from build123d import *

# Parameters (mm, degrees)
BOSS_EXTRUDE1_DEPTH = 38.1


with BuildPart() as part:
    # Sketch1 → Boss-Extrude1 (new body)
    with BuildSketch(Plane.XY):
        with BuildLine():
            Line((88.9, -50.8), (88.9, 50.8))
            ThreePointArc((88.9, 50.8), (57.095135122, 42.185130239), (25.4, 51.195336702))
            ThreePointArc((25.4, 51.195336702), (-57.15, 0), (25.4, -51.195336702))
            ThreePointArc((25.4, -51.195336702), (57.095135122, -42.185130239), (88.9, -50.8))
        make_face()
        with BuildLine():
            ThreePointArc((82.55, -40.628164989), (54.413891048, -35.903084421), (26.818032813, -43.144328898))
            ThreePointArc((26.818032813, -43.144328898), (24.611630749, -44.439932852), (22.342791686, -45.622797587))
            ThreePointArc((22.342791686, -45.622797587), (-50.735562995, 2.557859955), (26.818032813, 43.144328898))
            ThreePointArc((26.818032813, 43.144328898), (54.413891048, 35.903084421), (82.55, 40.628164989))
            Line((82.55, 40.628164989), (82.55, -40.628164989))
        make_face(mode=Mode.SUBTRACT)
    extrude(amount=BOSS_EXTRUDE1_DEPTH)


solid = part.part
Verification items for the finished model (mm, model axes). A direction names the side the tool comes from. Give positions to 0.01 mm unless a question says otherwise; leave off trailing zeros. Order: outer loops, then holes, each group sorted by start corner. A loop starts at its lowest first (then second) coordinate and runs counter-clockwise, first axis right, second up. Notation, with made-up numbers: M -12,-21.5 L 17,-21.5 A9 ccw 17,-16.5 Z; hole C 83,28.25 d9. An arc over 180 degrees is marked long. Use one line per item in the form item = value. Start each with the question number.
Q1. Section check B-B (x = 0). Enter the section's corners in (y, z).
Q2. Scan lines: line 1 along Y through (x, z) = (0, 8); line 2 along X through (y, z) = (3, 24); line 3 along Y through (x, z) = (67.5, 19.5). Record each from-to range of solid material in increasing order. Write a range as [from, to].
Q3. Access from +Z, -Z, +X, -X, +Y, -Y to the whole of each face (thin tool, end or side, straight path). Record for faces 4 (the cylindrical face through (56.63, -42.19, 18.78)), 5 (the flat face through (82.55, 1, 19)).
Q4. Section check A-A (y = 0). Enter the section's corners in (x, z), then the cut area to 3 significant figures.
Q5. Section check D-D (z = 5.5). Enter the section's corners in (x, y), then the cut area to 3 significant figures.
Q6. Section check C-C (y = 48.5). Enter the section's corners in (x, z).
Q7. Mould release check, pull along Z, two halves, no side actions. Record for faces 1 (the cylindrical face through (-57.127, 1.625, 18.783)), 2 (the flat face through (32, -42, 0)), 3 (the flat face through (32, -42, 38.1)): +Z half, -Z half, draft (parallel to the pull), parting line (faces both ways), or undercut.
Q8. Go/stop test with flat-tipped pins: pin 1 Ø8 at (x, z) = (74, 32.5) entering from +Y; pin 2 Ø1.5 at (x, z) = (18, 5.5) entering from -Y. Record where each tip stops, or that it passes through.
Evaluation:
q1.outline = M -57.15,0 L -50.8,0 L -50.8,38.1 L -57.15,38.1 Z; M 50.8,0 L 57.15,0 L 57.15,38.1 L 50.8,38.1 Z
q2.line_1 = [-57.15, -50.8], [50.8, 57.15]
q2.line_2 = [-57.07, -50.71], [82.55, 88.9]
q2.line_3 = [-43, -36.58], [36.58, 43]
q3.face_4 = +Z, -Z, -Y
q3.face_5 = +Z, -Z
q4.outline = M -57.15,0 L -50.8,0 L -50.8,38.1 L -57.15,38.1 Z; M 82.55,0 L 88.9,0 L 88.9,38.1 L 82.55,38.1 Z
q4.area = 484 mm2
q5.outline = M 25.4,-51.2 A61.6 cw 88.9,-50.8 L 88.9,50.8 A61.6 cw 25.4,51.2 A57.15 ccw long Z; hole M 26.82,-43.14 A67.95 cw 82.55,-40.63 L 82.55,40.63 A67.95 cw 26.82,43.14 A50.8 ccw long Z
q5.area = 2,790 mm2
q6.outline = M -30.23,0 L -15.11,0 L -15.11,38.1 L -30.23,38.1 Z; M 15.11,0 L 30.31,0 L 30.31,38.1 L 15.11,38.1 Z; M 84.65,0 L 88.9,0 L 88.9,38.1 L 84.65,38.1 Z
q7.face_1 = draft
q7.face_2 = -Z half
q7.face_3 = +Z half
q8.pin_1 = 45.7
q8.pin_2 = -54.48
